CAD build for the part. Positions are in the model's coordinates, mm. Face numbers are marked on the shaded views. Round coordinates to 2 decimals unless told otherwise and drop trailing zeros. Loops run counter-clockwise (first coordinate to the right, second up) from the corner with the lowest first, then second, coordinate; pieces in that order, holes last. Notation, with made-up numbers: M -0.5,37 L 32.5,37 A27 ccw 32.5,72 Z; hole C 14.25,0 d4. An arc over 180 degrees is marked long. Use a Markdown table: item, result. Add a question column.
(1) Band-saw the part on C-C, the plane y = -16. Write the cut outline in (x, z).
(2) Band-saw the part on D-D, the plane z = 38. Write the cut outline in (x, y), and give its area (3 significant figures).
(3) Two-plate mould, pull along X, no slides. Class the marked faces 1, 2 and 3: released by +X, released by -X, zero draft, split by the parting line, or undercut.
(4) Band-saw the part on A-A, the plane z = 10. Give the number of separate pieces and of enclosed holes in the cut face, and give its area (3 significant figures).
(5) Band-saw the part on B-B, the plane x = 18.5. Write the cut outline in (y, z), and give its area (3 significant figures).
(6) Wall check: L1, parallel to Y at x = 10.5, z = 38; L2, parallel to Y at x = -5.5, z = 43; L3, parallel to Z at x = -6.5, y = 9. Give the ranges that are in metal, low to high.
(7) Flat gauge pins, fed straight in: P1, Ø1, axis at y = 26, z = 43, coming from the -X side; P2, Ø6, axis at x = -1.5, y = -9, coming from the +Z side; P3, Ø3, axis at x = 24, z = 35.5, coming from the -Y side. Where does each tip first touch, or does it go through?
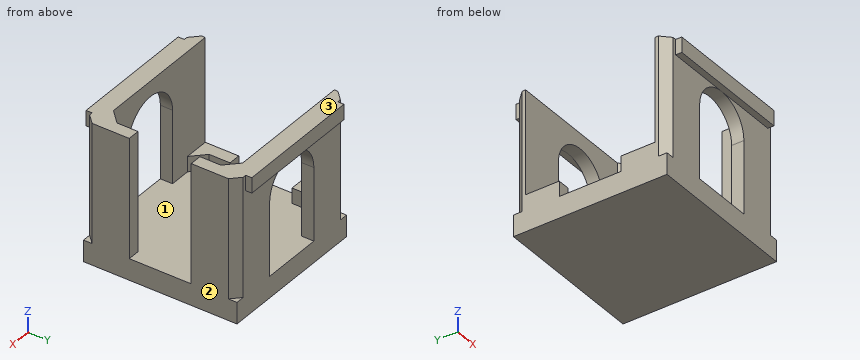
from build123d import *

# Parameters (mm, degrees)
SKETCH_W     = 50.3
SKETCH_H     = 50.3
PAD_DEPTH    = 7
PAD001_DEPTH = 39
SKETCH002_W  = 42.3
SKETCH002_H  = 34
POCKET_DEPTH = 15
SKETCH003_W  = 42.3
SKETCH003_H  = 6
PAD002_DEPTH = 5
PAD003_DEPTH = 4
PAD004_DEPTH = 4


with BuildPart() as part:
    # Sketch → Pad (new body)
    with BuildSketch(Plane.XY):
        Rectangle(SKETCH_W, SKETCH_H)
    extrude(amount=PAD_DEPTH)

    # Sketch001 (on Face6 of Pad) → Pad001 (join)
    with BuildSketch(Plane.XY.offset(7)):
        Polygon((17, 21.15), (21.15, 17), (21.15, 10.15), (25.15, 10.15), (25.15, 22.321573), (22.321573, 25.15), (10.15, 25.15), (10.15, 21.15), align=None)
        Polygon((-17, 21.15), (-21.15, 17), (-21.15, 10.15), (-25.15, 10.15), (-25.15, 22.321573), (-22.321573, 25.15), (-10.15, 25.15), (-10.15, 21.15), align=None)
        Polygon((17, -21.15), (21.15, -17), (21.15, -10.15), (25.15, -10.15), (25.15, -22.321573), (22.321573, -25.15), (10.15, -25.15), (10.15, -21.15), align=None)
        Polygon((-17, -21.15), (-21.15, -17), (-21.15, -10.15), (-25.15, -10.15), (-25.15, -22.321573), (-22.321573, -25.15), (-10.15, -25.15), (-10.15, -21.15), align=None)
    extrude(amount=PAD001_DEPTH)

    # Sketch002 (on Face13 of Pad001) → Pocket (cut)
    with BuildSketch(Plane(origin=(-25.15, 0, 0), x_dir=(0, -1, 0), z_dir=(-1, 0, 0))):
        with Locations((0, 29)):
            Rectangle(SKETCH002_W, SKETCH002_H)
    extrude(amount=-POCKET_DEPTH, mode=Mode.SUBTRACT)

    # Sketch003 (on Face50 of Pocket) → Pad002 (join)
    with BuildSketch(Plane.XY.offset(46)):
        with Locations((0, -24.15)):
            Rectangle(SKETCH003_W, SKETCH003_H)
        with Locations((0, 24.15)):
            Rectangle(SKETCH003_W, SKETCH003_H)
    extrude(amount=-PAD002_DEPTH)

    # Sketch004 (on Face44 of Pad002) → Pad003 (join)
    with BuildSketch(Plane.XZ.offset(25.15)):
        with BuildLine():
            ThreePointArc((10.15, 30.85), (0, 41), (-10.15, 30.85))
            Line((-10.15, 41.1), (-10.15, 30.85))
            Line((10.15, 41.1), (-10.15, 41.1))
            Line((10.15, 30.85), (10.15, 41.1))
        make_face()
    extrude(amount=-PAD003_DEPTH)

    # Sketch005 (on Face6 of Pad003) → Pad004 (join)
    with BuildSketch(Plane(origin=(0, 25.15, 0), x_dir=(-1, 0, 0), z_dir=(0, 1, 0))):
        with BuildLine():
            ThreePointArc((10.15, 30.85), (0, 41), (-10.15, 30.85))
            Line((-10.15, 30.85), (-10.15, 41.1))
            Line((-10.15, 41.1), (10.15, 41.1))
            Line((10.15, 30.85), (10.15, 41.1))
        make_face()
    extrude(amount=-PAD004_DEPTH)


solid = part.part
Return value:
| question | item | result |
|---|---|---|
| 1 | outline | M -25.15,0 L 25.15,0 L 25.15,46 L 21.15,46 L 21.15,7 L -21.15,7 L -21.15,12 L -25.15,12 Z |
| 2 | outline | M -25.15,-22.32 L -22.32,-25.15 L -7.2,-25.15 L -7.2,-21.15 L -25.15,-21.15 Z; M -25.15,21.15 L -7.2,21.15 L -7.2,25.15 L -22.32,25.15 L -25.15,22.32 Z; M 7.2,-25.15 L 22.32,-25.15 L 25.15,-22.32 L 25.15,-10.15 L 21.15,-10.15 L 21.15,-17 L 17,-21.15 L 7.2,-21.15 Z; M 7.2,21.15 L 17,21.15 L 21.15,17 L 21.15,10.15 L 25.15,10.15 L 25.15,22.32 L 22.32,25.15 L 7.2,25.15 Z |
| 2 | area | 376 mm^2 |
| 3 | face 1 | undercut |
| 3 | face 2 | released by +X |
| 3 | face 3 | zero draft |
| 4 | separate pieces | 4 |
| 4 | enclosed holes | 0 |
| 4 | area | 434 mm^2 |
| 5 | outline | M -27.15,41 L -25.15,41 L -25.15,0 L 25.15,0 L 25.15,41 L 27.15,41 L 27.15,46 L 19.65,46 L 19.65,7 L -19.65,7 L -19.65,46 L -27.15,46 Z |
| 5 | area | 801 mm^2 |
| 6 | L1 | -25.15 to -21.15, 21.15 to 25.15 |
| 6 | L2 | -27.15 to -21.15, 21.15 to 27.15 |
| 6 | L3 | 0 to 7 |
| 7 | P1 | x = -21.15 |
| 7 | P2 | z = 7 |
| 7 | P3 | y = -24.97 |
